Check sheet for the drawn part. Datum: minimum x, y, z corner. Units: mm. A direction names the side the tool comes from. Round coordinates to 2 decimals unless told otherwise and drop trailing zeros. Write each loop counter-clockwise with the first axis right and the second up, starting at its lowest first coordinate (ties: lowest second). Pieces come first, ordered by that corner, then holes. Notation, with made-up numbers: (-36, -1) -> (-26, -1) arc R32 ccw to (-26, 36) -> close; hole circle Ø1 at (-35, 39.5). An arc over 180 degrees is marked (long way). Use a Markdown table: item, result.
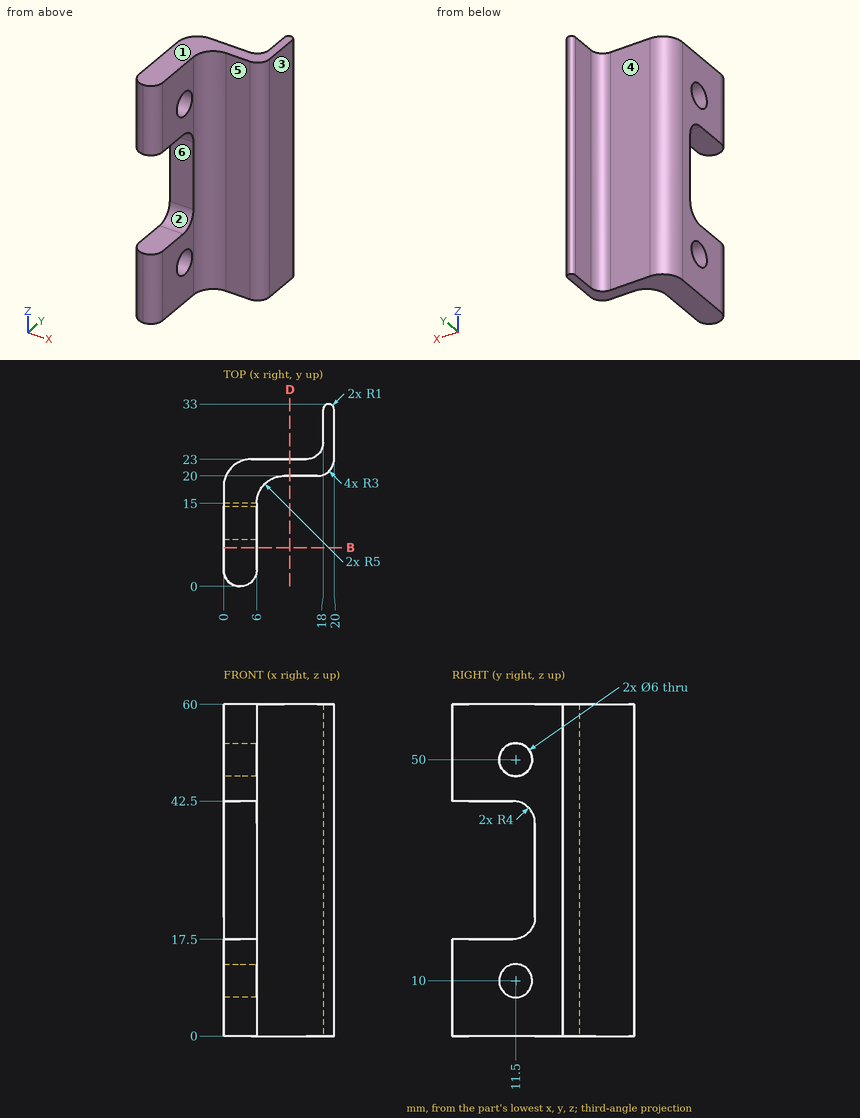
(1) Gauge pin test, flat ends, axial feed: pin 1 Ø10 at (y, z) = (24.5, 38.5) entering from -X; pin 2 Ø3 at (x, z) = (9, 30) entering from +Y; pin 3 Ø1.5 at (x, z) = (10.5, 48.5) entering from -Y. Record the tip position at first contact, or that the pin passes through.
A:
| item | result |
|---|---|
| pin 1 | stops at x = 0.23 |
| pin 2 | stops at y = 23 |
| pin 3 | stops at y = 19.84 |
(2) Section check B-B on y = 7. Record the cut outline in (x, z), plus the area to 3 significant figures.
A:
| item | result |
|---|---|
| outline | (0, 0) -> (6, 0) -> (6, 17.5) -> (0, 17.5) -> close; (0, 42.5) -> (6, 42.5) -> (6, 60) -> (0, 60) -> close |
| area | 210 mm2 |
(3) Access from +Z, -Z, +X, -X, +Y, -Y to the whole of each face (thin tool, end or side, straight path). Record for the marked faces 4, 5 and 6.
A:
| item | result |
|---|---|
| face 4 | +Z, -Z, -X, +Y |
| face 5 | +Z, -Z, +X, -Y |
| face 6 | +X, -X, -Y |
(4) Thickness scan on line 1 (Y direction, x = 3.15, z = 10) (1 decimal); line 2 (Y direction, x = 14, z = 6.5); line 3 (X direction, y = 26, z = 33.5). Record the ranges inside material, lowest first.
A:
| item | result |
|---|---|
| line 1 | y = 0 to 8.5, 14.5 to 22.6 |
| line 2 | y = 20 to 23 |
| line 3 | x = 18 to 20 |
(5) Release check for a two-part mould opening along Z. For the marked faces 1, 2 and 3 record: +Z half, -Z half, draft (parallel to the pull), parting line (faces both ways), or undercut.
A:
| item | result |
|---|---|
| face 1 | +Z half |
| face 2 | undercut |
| face 3 | draft |
(6) Section check D-D on x = 12. Record the cut outline in (y, z), plus the area to 3 significant figures.
A:
| item | result |
|---|---|
| outline | (20, 0) -> (23, 0) -> (23, 60) -> (20, 60) -> close |
| area | 180 mm2 |
